Model file for the job. Use its own axes, mm. Coordinates: 2 decimals unless noted, no trailing zeros. Loops run counter-clockwise (first coordinate to the right, second up) from the corner with the lowest first, then second, coordinate; pieces in that order, holes last.
from build123d import *

# Parameters (mm, degrees)
F0_W           = 95
F0_H           = 95
F1_DEPTH       = 4.5
F2_R           = 2.1
F3_DEPTH       = 4.5
F4_R           = 1
F6_D           = 3.3
F6_CSINK_D     = 6.72
F6_CSINK_ANGLE = 90


with BuildPart() as f1:
    # F0 (on Front) → F1 (new body)
    with BuildSketch(Plane.XZ):
        Rectangle(F0_W, F0_H)
    extrude(amount=F1_DEPTH)

    # F2 (on face) → F3 (cut, through all)
    with BuildSketch(Plane.XZ.offset(4.5)):
        with Locations((43.5, 43.5)):
            Circle(F2_R)
        with Locations((43.5, -43.5)):
            Circle(F2_R)
        with Locations((-32.5, -43.5)):
            Circle(F2_R)
        with Locations((-43.5, 43.5)):
            Circle(F2_R)
    extrude(amount=-F3_DEPTH, mode=Mode.SUBTRACT)

    # F4
    f4_edges = [f1.edges().sort_by_distance(p)[0] for p in [
        (-47.5, -2.25, 47.5),
        (47.5, -2.25, 47.5),
        (47.5, -2.25, -47.5),
        (-47.5, -2.25, -47.5),
    ]]
    fillet(f4_edges, radius=F4_R)

    # F6 (through all)
    with Locations(Plane(origin=(0, 0, 0), x_dir=(-1, 0, 0), z_dir=(0, 1, 0))):
        with Locations((-39.5, 30.2), (36.7, 30.2), (36.7, -29.2), (-39.5, -29.2)):
            CounterSinkHole(F6_D / 2, F6_CSINK_D / 2, counter_sink_angle=F6_CSINK_ANGLE)


solid = f1.part
Q1. Slice it at C-C (z = 43.5). List the corners of the cut face in (x, y).
Answers:
outline: (-47.5, -4.5) - (-45.6, -4.5) - (-45.6, 0) - (-47.5, 0) - close; (-41.4, -4.5) - (41.4, -4.5) - (41.4, 0) - (-41.4, 0) - close; (45.6, -4.5) - (47.5, -4.5) - (47.5, 0) - (45.6, 0) - close
Q2. Slice it at B-B (x = -36.7). List the corners of the cut face in (y, z).
Answers:
outline: (-4.5, -47.5) - (0, -47.5) - (0, -32.56) - (-1.71, -30.85) - (-4.5, -30.85) - close; (-4.5, -27.55) - (-1.71, -27.55) - (0, -25.84) - (0, 26.84) - (-1.71, 28.55) - (-4.5, 28.55) - close; (-4.5, 31.85) - (-1.71, 31.85) - (0, 33.56) - (0, 47.5) - (-4.5, 47.5) - close
Q3. Mould opens along X. For faces 1 (the flat face through (-47.5, -2, -1)), 2 (the cylindrical face through (43.04, -2.28, -45.55)), 3 (the flat face through (-1, 0, 1)), 4 (the cylindrical face through (-35.176, -3.125, -29.832)) say: +X half, -X half, draft (parallel to the pull), parting line (faces both ways), or undercut.
Answers:
face 1: -X half
face 2: undercut
face 3: draft
face 4: undercut
Q4. Slice it at A-A (z = -29.2). List the corners of the cut face in (x, y), and give its area (3 significant figures).
Answers:
outline: (-47.5, -4.5) - (-38.35, -4.5) - (-38.35, -1.71) - (-40.06, 0) - (-47.5, 0) - close; (-35.05, -4.5) - (37.85, -4.5) - (37.85, -1.71) - (36.14, 0) - (-33.34, 0) - (-35.05, -1.71) - close; (41.15, -4.5) - (47.5, -4.5) - (47.5, 0) - (42.86, 0) - (41.15, -1.71) - close
area: 392 mm2
Q5. Drill centre lines: line 1 (X direction, y = -2.6, z = -29.2); line 2 (Z direction, x = -36.7, y = -2.45); line 3 (Z direction, x = 43.5, y = -0.9). Where is each one in solid material? Low to high.
Answers:
line 1: x = -47.5 to -38.35, -35.05 to 37.85, 41.15 to 47.5
line 2: z = -47.5 to -30.85, -27.55 to 28.55, 31.85 to 47.5
line 3: z = -47.5 to -45.6, -41.4 to 41.4, 45.6 to 47.5
